Check sheet for the modelled part. Datum: model origin and axes. Units: mm. A direction names the side the tool comes from. Round coordinates to 2 decimals unless told otherwise and drop trailing zeros. Write each loop counter-clockwise with the first axis right and the second up, starting at its lowest first coordinate (ties: lowest second). Pieces come first, ordered by that corner, then holes.
Item 1: Cross-section at B-B on x = 121. Enter the section's corners in (y, z), plus the area to 3 significant figures.
Item 2: Material ranges on line 1 (Y direction, x = 401.5, z = 332); line 2 (Z direction, x = 249.5, y = 226), recorded low to high.
Item 3: Go/stop test with flat-tipped pins: pin 1 Ø10 at (x, z) = (411.5, 385.5) entering from +Y; pin 2 Ø6 at (y, z) = (6.5, 154) entering from -X; pin 3 Ø1.5 at (x, y) = (237, 47) entering from +Z. Record where each tip stops, or that it passes through.
Item 4: Tool access check on faces 1 (the flat face through (20, 410, 296)), 2 (the flat face through (10, 0, 296)), 3 (the flat face through (410, 420, 296)), 4 (the flat face through (10, 20, 296)). Record the directions out of +Z, -Z, +X, -X, +Y, -Y that give a thin tool (end or side, any length) a straight path to the whole face; none if there is none.
Item 5: Cross-section at A-A on z = 400.5. Enter the section's corners in (x, y), plus the area to 3 significant figures.
Item 6: Cross-section at D-D on z = 822. Enter the section's corners in (x, y), plus the area to 3 significant figures.
Item 7: Release check for a two-part mould opening along Y. For faces 5 (the flat face through (420, 10, 296)), 6 (the flat face through (410, 0, 296)), 7 (the flat face through (207, 430, 610)), 8 (the flat face through (410, 20, 296)) record: +Y half, -Y half, draft (parallel to the pull), parting line (faces both ways), or undercut.
Item 8: Cross-section at C-C on y = 62.5. Enter the section's corners in (x, z), plus the area to 3 significant figures.
from build123d import *

# Parameters (mm, degrees)
F0_W     = 20
F0_H     = 20
F1_DEPTH = 600
F2_W     = 440
F2_H     = 440
F3_DEPTH = 20
F4_W     = 440
F4_H     = 20
F5_DEPTH = 500
F6_R     = 20


with BuildPart() as f1:
    # F0 (on Top) → F1 (new body)
    with BuildSketch(Plane.XY):
        with Locations((10, 10)):
            Rectangle(F0_W, F0_H)
        with Locations((10, 410)):
            Rectangle(F0_W, F0_H)
        with Locations((410, 10)):
            Rectangle(F0_W, F0_H)
        with Locations((410, 410)):
            Rectangle(F0_W, F0_H)
    extrude(amount=F1_DEPTH)

    # F2 (on face) → F3 (join)
    with BuildSketch(Plane.XY.offset(600)):
        with Locations((210, 210)):
            Rectangle(F2_W, F2_H)
    extrude(amount=F3_DEPTH)

    # F4 (on face) → F5 (join)
    with BuildSketch(Plane.XY.offset(620)):
        with Locations((210, 0)):
            Rectangle(F4_W, F4_H)
    extrude(amount=F5_DEPTH)

    # F6
    f6_edges = [f1.edges().sort_by_distance(p)[0] for p in [
        (430, 0, 1120),
        (-10, 0, 1120),
    ]]
    fillet(f6_edges, radius=F6_R)


solid = f1.part
Response values:
1. outline: (-10, 600) - (430, 600) - (430, 620) - (10, 620) - (10, 1120) - (-10, 1120) - close
1. area: 18,800 mm2
2. line 1: y = 0 to 20, 400 to 420
2. line 2: z = 600 to 620
3. pin 1: stops at y = 420
3. pin 2: stops at x = 0
3. pin 3: stops at z = 620
4. face 1: -Z, +Y, -Y
4. face 2: -Z, +X, -X, -Y
4. face 3: -Z, +X, -X, +Y
4. face 4: -Z, +X, -X
5. outline: (0, 0) - (20, 0) - (20, 20) - (0, 20) - close; (0, 400) - (20, 400) - (20, 420) - (0, 420) - close; (400, 0) - (420, 0) - (420, 20) - (400, 20) - close; (400, 400) - (420, 400) - (420, 420) - (400, 420) - close
5. area: 1,600 mm2
6. outline: (-10, -10) - (430, -10) - (430, 10) - (-10, 10) - close
6. area: 8,800 mm2
7. face 5: draft
7. face 6: -Y half
7. face 7: +Y half
7. face 8: undercut
8. outline: (-10, 600) - (430, 600) - (430, 620) - (-10, 620) - close
8. area: 8,800 mm2
